Read the model definition and answer for the solid it produces. Units are mm, in the model's axes. Face numbers are marked on the shaded views. A direction names the side the tool comes from. Coordinates: 2 decimals unless noted, no trailing zeros. Write each loop counter-clockwise with the first axis right and the second up, starting at its lowest first coordinate (ties: lowest second). Pieces come first, ordered by that corner, then holes.
(1) Section C-C on y = 3.2 is taken. State how many separate pieces and enclosed holes the cut face has, then the cut area to 3 significant figures.
(2) The mould has two halves that part along Z. Classify the marked faces 4, 5 and 6: +Z half, -Z half, draft (parallel to the pull), parting line (faces both ways), or undercut.
(3) Section D-D on z = 7.1 is taken. Write down the section's boundary in (x, y).
(4) Section A-A on z = 2.25 is taken. Write down the section's boundary in (x, y) (3 decimals).
(5) Section B-B on x = -4.8 is taken. Write down the section's boundary in (y, z) (3 decimals).
(6) Find the intervals of material crossed by probe 1 along X at (y, z) = (2.75, 2.25) (3 decimals); probe 2 along Z at (x, y) = (9, 2.5); probe 3 along Y at (x, z) = (-7.75, 7.1), in increasing order.
(7) Given pin 1 (3 mm diameter, centred on x = 21, y = 4.5, fed in from +Z); pin 2 (0.5 mm diameter, centred on x = 8, z = 6, fed in from -Y); pin 3 (3.5 mm diameter, centred on y = 3, z = 7.5, fed in from +X); pin 4 (3 mm diameter, centred on x = 0.5, y = 2.5, fed in from +Z), each flat-ended and moving along its own axis, determine where each tip first touches the part or whether it passes through.
(8) Which of the six approach directions +Z, -Z, +X, -X, +Y, -Y give full straight-line access (tool end or side, diameter ignored) to the marked faces 1, 2 and 3?
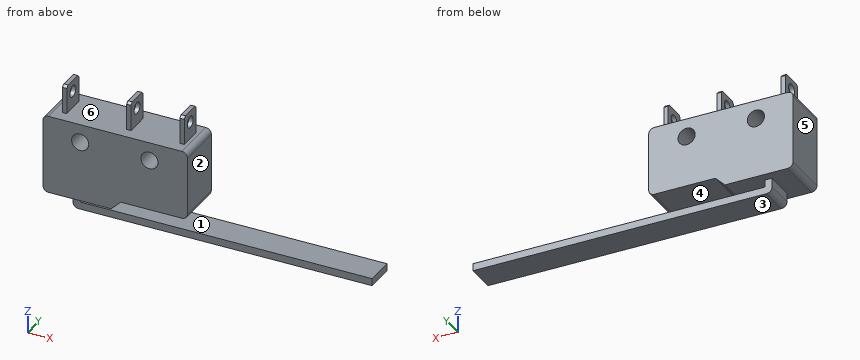
from build123d import *

# Parameters (mm, degrees)
SKETCH1_W           = 19.8
SKETCH1_H           = 9.5
BOSS_EXTRUDE1_DEPTH = 6.4
SKETCH2_W           = 10.65
SKETCH2_H           = 6.4
BOSS_EXTRUDE2_DEPTH = 1.3
CHAMFER3_SIZE       = 1.3
FILLET1_R           = 0.75
SKETCH3_W           = 1
SKETCH3_H           = 4
BOSS_EXTRUDE3_DEPTH = 2
SKETCH4_W           = 1
SKETCH4_H           = 4
BOSS_EXTRUDE4_DEPTH = 40
FILLET2_R           = 0.75
SKETCH5_R           = 1.175
CUT_EXTRUDE1_DEPTH  = 6.4
SKETCH6_W           = 0.6
SKETCH6_H           = 3.2
BOSS_EXTRUDE5_DEPTH = 3.9
SKETCH8_R           = 0.8
CUT_EXTRUDE2_DEPTH  = 16.7
CHAMFER4_SIZE       = 0.33


with BuildPart() as part:
    # Sketch1 → Boss-Extrude1 (new body)
    with BuildSketch(Plane(origin=(0, 0, 0), x_dir=(1, 0, 0), z_dir=(0, 1, 0))):
        Rectangle(SKETCH1_W, SKETCH1_H)
    extrude(amount=BOSS_EXTRUDE1_DEPTH)

    # Sketch2 → Boss-Extrude2 (add)
    with BuildSketch(Plane(origin=(0, 0, -4.75), x_dir=(-1, 0, 0), z_dir=(0, 0, -1))):
        with Locations((4.575, 3.2)):
            Rectangle(SKETCH2_W, SKETCH2_H)
    extrude(amount=BOSS_EXTRUDE2_DEPTH)

    # Chamfer3
    chamfer3_edges = [part.edges().sort_by_distance(p)[0] for p in [
        (0.75, 3.2, -6.05),
    ]]
    chamfer(chamfer3_edges, length=CHAMFER3_SIZE - 0.0001)  # a hair under: the kernel refuses the full size

    # Fillet1
    fillet1_edges = [part.edges().sort_by_distance(p)[0] for p in [
        (-9.9, 3.2, -6.05),
        (9.9, 3.2, 4.75),
        (-9.9, 3.2, 4.75),
        (9.9, 3.2, -4.75),
    ]]
    fillet(fillet1_edges, radius=FILLET1_R)

    # Sketch3 → Boss-Extrude3 (add)
    with BuildSketch(Plane(origin=(0, 0, -6.05), x_dir=(-1, 0, 0), z_dir=(0, 0, -1))):
        with Locations((5.9, 3.2)):
            Rectangle(SKETCH3_W, SKETCH3_H)
    extrude(amount=BOSS_EXTRUDE3_DEPTH)

    # Sketch4 → Boss-Extrude4 (add)
    with BuildSketch(Plane(origin=(-5.4, 0, 0), x_dir=(0, 0, -1), z_dir=(1, 0, 0))):
        with Locations((7.55, 3.2)):
            Rectangle(SKETCH4_W, SKETCH4_H)
    extrude(amount=BOSS_EXTRUDE4_DEPTH)

    # Fillet2
    fillet2_edges = [part.edges().sort_by_distance(p)[0] for p in [
        (-6.4, 3.2, -8.05),
    ]]
    fillet(fillet2_edges, radius=FILLET2_R)

    # Sketch5 → Cut-Extrude1 (cut)
    with BuildSketch(Plane(origin=(0, 6.4, 0), x_dir=(1, 0, 0), z_dir=(0, 1, 0))):
        with Locations(Location((-4.8, -2.25, 0), (0, 0, 270))):
            Circle(SKETCH5_R)
        with Locations(Location((4.7, -2.25, 0), (0, 0, 270))):
            Circle(SKETCH5_R)
    extrude(amount=-CUT_EXTRUDE1_DEPTH, mode=Mode.SUBTRACT)

    # Sketch6 → Boss-Extrude5 (add)
    with BuildSketch(Plane.XY.offset(4.75)):
        with Locations((-7.75, 3.2)):
            Rectangle(SKETCH6_W, SKETCH6_H)
        with Locations((1.05, 3.2)):
            Rectangle(SKETCH6_W, SKETCH6_H)
        with Locations((8.35, 3.2)):
            Rectangle(SKETCH6_W, SKETCH6_H)
    extrude(amount=BOSS_EXTRUDE5_DEPTH)

    # Sketch8 → Cut-Extrude2 (cut)
    with BuildSketch(Plane.ZY.offset(8.05)):
        with Locations((7.1, 3.2)):
            Circle(SKETCH8_R)
    extrude(amount=-CUT_EXTRUDE2_DEPTH, mode=Mode.SUBTRACT)

    # Chamfer4
    chamfer4_edges = [part.edges().sort_by_distance(p)[0] for p in [
        (-7.75, 1.6, 8.65),
        (-7.75, 4.8, 8.65),
        (1.05, 1.6, 8.65),
        (1.05, 4.8, 8.65),
        (8.35, 1.6, 8.65),
        (8.35, 4.8, 8.65),
    ]]
    chamfer(chamfer4_edges, length=CHAMFER4_SIZE)


solid = part.part
Response:
1. separate pieces: 4
1. enclosed holes: 2
1. area: 238 mm2
2. face 4: undercut
2. face 5: draft
2. face 6: +Z half
3. outline: (-8.05, 1.6) - (-7.45, 1.6) - (-7.45, 2.4) - (-8.05, 2.4) - close; (-8.05, 4) - (-7.45, 4) - (-7.45, 4.8) - (-8.05, 4.8) - close; (0.75, 1.6) - (1.35, 1.6) - (1.35, 2.4) - (0.75, 2.4) - close; (0.75, 4) - (1.35, 4) - (1.35, 4.8) - (0.75, 4.8) - close; (8.05, 1.6) - (8.65, 1.6) - (8.65, 2.4) - (8.05, 2.4) - close; (8.05, 4) - (8.65, 4) - (8.65, 4.8) - (8.05, 4.8) - close
4. outline: (-9.9, 0) - (-5.975, 0) - (-5.975, 6.4) - (-9.9, 6.4) - close; (-3.625, 0) - (3.525, 0) - (3.525, 6.4) - (-3.625, 6.4) - close; (5.875, 0) - (9.9, 0) - (9.9, 6.4) - (5.875, 6.4) - close
5. outline: (0, -6.05) - (6.4, -6.05) - (6.4, 1.075) - (0, 1.075) - close; (0, 3.425) - (6.4, 3.425) - (6.4, 4.75) - (0, 4.75) - close; (1.2, -8.05) - (5.2, -8.05) - (5.2, -7.05) - (1.2, -7.05) - close
6. probe 1: x = -9.9 to -5.975, -3.625 to 3.525, 5.875 to 9.9
6. probe 2: z = -8.05 to -7.05, -4.75 to 4.75
6. probe 3: y = 1.6 to 2.4, 4 to 4.8
7. pin 1: stops at z = -7.05
7. pin 2: stops at y = 1.6
7. pin 3: stops at x = 8.65
7. pin 4: stops at z = 8.65
8. face 1: +X, +Y, -Y
8. face 2: +Z, +X, +Y, -Y
8. face 3: -Z, +X, -X, +Y, -Y
